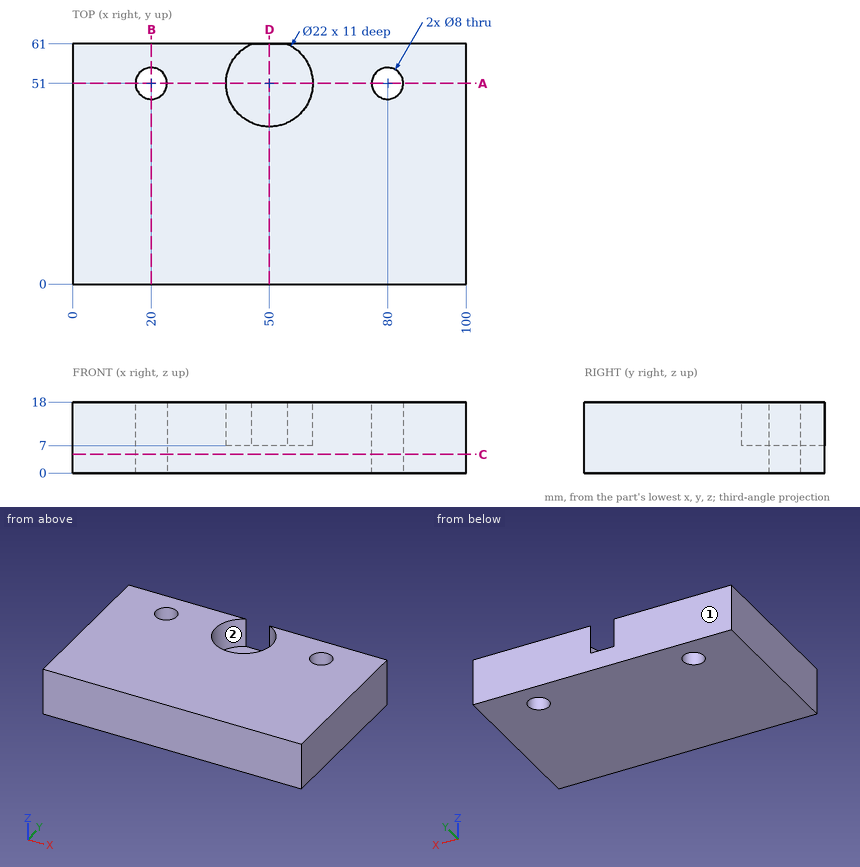
Design review of the part shown in the three views and the two pictorial views. Dimensions are in mm from the part's minimum x, y and z. A direction names the side the tool comes from. Round coordinates to 2 decimals unless told otherwise and drop trailing zeros. Write each loop counter-clockwise with the first axis right and the second up, starting at its lowest first coordinate (ties: lowest second). Pieces come first, ordered by that corner, then holes. Notation, with made-up numbers: M -24.5,16 L -9.5,16 A14 cw -9.5,33 Z; hole C -37.75,27.25 d9. An arc over 180 degrees is marked long. One line per item, written item: value. Start each with the question number.
1. To check wall thickness, follow probe 1 along Y at (x, z) = (80, 8.5); probe 2 along X at (y, z) = (51.5, 6.5); probe 3 along Y at (x, z) = (41.5, 17). State the ranges of each line that lie inside material, in increasing order. Write a range as from..to.
2. Take a section at C-C on z = 4.75. State the section outline as (x, y) points, then the cut area to 3 significant figures.
3. Take a section at A-A on y = 51. State the section outline as (x, z) points, then the cut area to 3 significant figures.
4. Clearance check with flat-ended pins moving along their axes: P1, Ø6, axis at y = 27, z = 8, coming from the -X side; P2, Ø20, axis at x = 50, y = 51, coming from the +Z side. State where each tip first meets the part, or that it passes through.
5. Take a section at B-B on x = 20. State the section outline as (y, z) points, then the cut area to 3 significant figures.
6. Take a section at D-D on x = 50. State the section outline as (y, z) points, then the cut area to 3 significant figures.
7. For the marked faces 1 and 2, list the 3-axis set-ups (+Z, -Z, +X, -X, +Y, -Y) from which the entire face can be reached by the end or side of a thin tool; tool diameter is ignored.
Computed:
1. probe 1: y = 0..47, 55..61
1. probe 2: x = 0..16.03, 23.97..76.03, 83.97..100
1. probe 3: y = 0..44.02, 57.98..61
2. outline: M 0,0 L 100,0 L 100,61 L 0,61 Z; hole C 20,51 d8; hole C 80,51 d8
2. area: 6,000 mm²
3. outline: M 0,0 L 16,0 L 16,18 L 0,18 Z; M 24,0 L 76,0 L 76,18 L 61,18 L 61,7 L 39,7 L 39,18 L 24,18 Z; M 84,0 L 100,0 L 100,18 L 84,18 Z
3. area: 1,270 mm²
4. P1: stops at x = 0
4. P2: stops at z = 7
5. outline: M 0,0 L 47,0 L 47,18 L 0,18 Z; M 55,0 L 61,0 L 61,18 L 55,18 Z
5. area: 954 mm²
6. outline: M 0,0 L 61,0 L 61,7 L 40,7 L 40,18 L 0,18 Z
6. area: 867 mm²
7. face 1: +Z, -Z, +X, -X, +Y
7. face 2: +Z
